For this review, take the finished solid that the model builds, in its own axes (mm). A direction names the side the tool comes from. Round coordinates to 2 decimals unless told otherwise and drop trailing zeros. Order: outer loops, then holes, each group sorted by start corner. A loop starts at its lowest first (then second) coordinate and runs counter-clockwise, first axis right, second up. Notation, with made-up numbers: M 47.5,43 L 75.5,43 A16 ccw 75.5,54 Z; hole C 68,6.25 d9. An arc over 180 degrees is marked long. Use a Markdown table: item, result.
from build123d import *

# Parameters (mm, degrees)
CROQUIS1_R              = 12.5
SALIENTE_EXTRUIR1_DEPTH = 10
CROQUIS2_W              = 55
CROQUIS2_H              = 10
SALIENTE_EXTRUIR2_DEPTH = 30


with BuildPart() as part:
    # Croquis1 → Saliente-Extruir1 (new body)
    with BuildSketch(Plane.XY):
        Polygon((0, 98.1), (27.5, 98.1), (27.5, 0), (-27.5, 0), (-27.5, 98.1), align=None)
        with Locations((0, 60)):
            Circle(CROQUIS1_R, mode=Mode.SUBTRACT)
    extrude(amount=SALIENTE_EXTRUIR1_DEPTH)

    # Croquis2 → Saliente-Extruir2 (add)
    with BuildSketch(Plane.XY.offset(10)):
        with Locations((0, 5)):
            Rectangle(CROQUIS2_W, CROQUIS2_H)
    extrude(amount=SALIENTE_EXTRUIR2_DEPTH)


solid = part.part
Q1. Wall thickness on line 1 along Y through (x, z) = (0, 3.25); line 2 along Y through (x, z) = (-21, 19): over which ranges is each line inside the solid? List them lowest first. Write a range as [from, to].
Determined:
| item | result |
|---|---|
| line 1 | y = [0, 47.5], [72.5, 98.1] |
| line 2 | y = [0, 10] |
Q2. Add section C-C (z = 7). Write out the cut boundary in (x, y).
Determined:
| item | result |
|---|---|
| outline | M -27.5,0 L 27.5,0 L 27.5,98.1 L -27.5,98.1 Z; hole C 0,60 d25 |
Q3. Add section B-B (y = 60). Write out the cut boundary in (x, z).
Determined:
| item | result |
|---|---|
| outline | M -27.5,0 L -12.5,0 L -12.5,10 L -27.5,10 Z; M 12.5,0 L 27.5,0 L 27.5,10 L 12.5,10 Z |
Q4. Add section A-A (x = 0). Write out the cut boundary in (y, z), then the cut area to 3 significant figures.
Determined:
| item | result |
|---|---|
| outline | M 0,0 L 47.5,0 L 47.5,10 L 10,10 L 10,40 L 0,40 Z; M 72.5,0 L 98.1,0 L 98.1,10 L 72.5,10 Z |
| area | 1,030 mm^2 |
Q5. Draft analysis for pull direction X (two halves, no side actions). For faces 3 (the cylindrical face through (-1.627, 72.394, 4.93)), 4 (the flat face through (0, 0, 20)), 5 (the flat face through (-27.5, 37.9, 9.5)), state which applies: pulls with the +X half, pulls with the -X half, needs draft (parallel to the pull), parting line crosses it, or undercut.
Determined:
| item | result |
|---|---|
| face 3 | undercut |
| face 4 | needs draft |
| face 5 | pulls with the -X half |
Q6. Machinability: for faces 1 (the flat face through (0, 98.1, 5)), 2 (the flat face through (0, 10, 25)), which of the approach directions +Z, -Z, +X, -X, +Y, -Y give a long, thin tool a straight path to every point of the face, cutting with its end or side? Answer none if there is none.
Determined:
| item | result |
|---|---|
| face 1 | +Z, -Z, +X, -X, +Y |
| face 2 | +Z, +X, -X, +Y |
Q7. Clearance check with flat-ended pins moving along their axes: pin 1 (4 mm diameter, centred on x = -12.5, z = 31.5, fed in from +Y); pin 2 (16.5 mm diameter, centred on x = -8.5, y = 41, fed in from +Z). State where each tip first meets the part, or that it passes through.
Determined:
| item | result |
|---|---|
| pin 1 | stops at y = 10 |
| pin 2 | stops at z = 10 |
Q8. Add section D-D (x = -7.5). Write out the cut boundary in (y, z), then the cut area to 3 significant figures.
Determined:
| item | result |
|---|---|
| outline | M 0,0 L 50,0 L 50,10 L 10,10 L 10,40 L 0,40 Z; M 70,0 L 98.1,0 L 98.1,10 L 70,10 Z |
| area | 1,080 mm^2 |
